from build123d import *

# Parameters (mm, degrees)
SKETCH_1_R          = 2.025
EXTRUDE_1_DEPTH     = 5
FILLET_1_R          = 2
SKETCH_2_R          = 5
CUT_EXTRUDE_1_DEPTH = 5


with BuildPart() as part:
    # 草图1 → 凸台-拉伸1 (new body)
    with BuildSketch(Plane(origin=(0, 0, 0), x_dir=(1, 0, 0), z_dir=(0, 1, 0))):
        with BuildLine():
            Line((7.5, 11.5), (-7.5, 11.5))
            ThreePointArc((-7.5, 11.5), (-12.096194078, 9.596194078), (-14, 5))
            Line((-14, 5), (-14, -15.546331524))
            Line((-14, -15.546331524), (26, -15.546331524))
            Line((26, -15.546331524), (14, -2.218981346))
            Line((14, -2.218981346), (14, 5))
            ThreePointArc((14, 5), (12.096194078, 9.596194078), (7.5, 11.5))
        make_face()
        with Locations((-7.5, -5)):
            Circle(SKETCH_1_R, mode=Mode.SUBTRACT)
        with Locations((7.5, -5)):
            Circle(SKETCH_1_R, mode=Mode.SUBTRACT)
        with Locations((-7.5, 5)):
            Circle(SKETCH_1_R, mode=Mode.SUBTRACT)
        with Locations((7.5, 5)):
            Circle(SKETCH_1_R, mode=Mode.SUBTRACT)
    extrude(amount=EXTRUDE_1_DEPTH)

    # 圆角1
    fillet_1_edges = [part.edges().sort_by_distance(p)[0] for p in [
        (14, 2.5, 2.218981346),
        (26, 2.5, 15.546331524),
        (-14, 2.5, 15.546331524),
    ]]
    fillet(fillet_1_edges, radius=FILLET_1_R)

    # 草图2 → 切除-拉伸1 (cut)
    with BuildSketch(Plane(origin=(0, 5, 0), x_dir=(1, 0, 0), z_dir=(0, 1, 0))):
        Circle(SKETCH_2_R)
    extrude(amount=-CUT_EXTRUDE_1_DEPTH, mode=Mode.SUBTRACT)


solid = part.part
Source: CAD feature listing. Evaluate the final solid. Frame: model axes, mm. A direction names the side the tool comes from. Coordinates: 2 decimals unless noted, no trailing zeros. Loops run counter-clockwise (first coordinate to the right, second up) from the corner with the lowest first, then second, coordinate; pieces in that order, holes last. Notation, with made-up numbers: M -37.5,47.5 L 13.5,47.5 A16 ccw 13.5,60.5 Z; hole C 49.25,44 d11. An arc over 180 degrees is marked long. Answer in a Markdown table with one row per item.
Q1. Draft query along X for faces 1 (the cylindrical face through (-12.045, 2.465, -9.646)), 2 (the flat face through (18.81, 2.46, 7.56)), 3 (the cylindrical face through (-9.11, 2.46, -3.77)), 4 (the flat face through (0, 2, -11.5)). Return one class per face: pulls with the +X half, pulls with the -X half, needs draft (parallel to the pull), parting line crosses it, or undercut.
Answers below:
| item | result |
|---|---|
| face 1 | pulls with the -X half |
| face 2 | pulls with the +X half |
| face 3 | undercut |
| face 4 | needs draft |
Q2. Section A-A on x = 0. Return the cut outline in (y, z).
Answers below:
| item | result |
|---|---|
| outline | M 0,-11.5 L 5,-11.5 L 5,-5 L 0,-5 Z; M 0,5 L 5,5 L 5,15.55 L 0,15.55 Z |
Q3. Set-up query: faces 5 (the cylindrical face through (5.89, 2.46, 6.23)), 6 (the flat face through (14, 2, -2)). Return all of +Z, -Z, +X, -X, +Y, -Y with unobstructed straight access to the full face (end or side cutting, diameter ignored); none if empty.
Answers below:
| item | result |
|---|---|
| face 5 | +Y, -Y |
| face 6 | -Z, +X, +Y, -Y |
Q4. Section D-D on z = 0. Return the cut outline in (x, y).
Answers below:
| item | result |
|---|---|
| outline | M -14,0 L -5,0 L -5,5 L -14,5 Z; M 5,0 L 14,0 L 14,5 L 5,5 Z |
Q5. Section B-B on y = 3.15. Return the cut outline in (x, z) (3 decimals).
Answers below:
| item | result |
|---|---|
| outline | M -14,-5 A6.5 ccw -7.5,-11.5 L 7.5,-11.5 A6.5 ccw 14,-5 L 14,1.451 A2 cw 14.514,2.79 L 22.994,12.208 A2 ccw 21.508,15.546 L -12,15.546 A2 ccw -14,13.546 Z; hole C -7.5,-5 d4.05; hole C -7.5,5 d4.05; hole C 0,0 d10; hole C 7.5,-5 d4.05; hole C 7.5,5 d4.05 |
Q6. First-contact query: pin 1 (2.5 mm diameter, centred on y = 3, z = -1, fed in from +X). Flat tip, straight axial feed; report the tip coordinate or a pass-through.
Answers below:
| item | result |
|---|---|
| pin 1 | stops at x = 14 |
Q7. Section C-C on z = 6.25. Return the cut outline in (x, y), plus the area to 3 significant figures.
Answers below:
| item | result |
|---|---|
| outline | M -14,0 L -9.09,0 L -9.09,5 L -14,5 Z; M -5.91,0 L 5.91,0 L 5.91,5 L -5.91,5 Z; M 9.09,0 L 17.63,0 L 17.63,5 L 9.09,5 Z |
| area | 126 mm^2 |
Q8. Ray query, probe 1 along Z at (x, y) = (7.5, 2.5) (3 decimals); probe 2 along X at (y, z) = (4, 0); probe 3 along Z at (x, y) = (-6, 3.7). Return the intervals inside material, ascending. Write a range as from..to.
Answers below:
| item | result |
|---|---|
| probe 1 | z = -11.5..-7.025, -2.975..2.975, 7.025..15.546 |
| probe 2 | x = -14..-5, 5..14 |
| probe 3 | z = -11.5..-6.36, -3.64..3.64, 6.36..15.55 |
